Verification items for the finished model (mm, model axes). Round coordinates to 2 decimals unless told otherwise and drop trailing zeros. Order: outer loops, then holes, each group sorted by start corner. A loop starts at its lowest first (then second) coordinate and runs counter-clockwise, first axis right, second up. Notation, with made-up numbers: M -36,-33.5 L 10,-33.5 A24 cw 10,-21.5 Z; hole C -13,-29 d2. An arc over 180 degrees is marked long. One line per item, written item: value. Start each with the question number.
from build123d import *

# Parameters (mm, degrees)
F0_W     = 40
F0_H     = 50
F1_DEPTH = 3
F3_D     = 4.1
F4_D     = 5.1
F5_R     = 5


with BuildPart() as f1:
    # F0 (on Front) → F1 (new body)
    with BuildSketch(Plane.XZ):
        Rectangle(F0_W, F0_H)
    extrude(amount=-F1_DEPTH)

    # F3 (through all)
    with Locations(Plane.XZ):
        with Locations((0, 15.5), (0, -15.5)):
            Hole(F3_D / 2)

    # F4 (through all)
    with Locations(Plane.XZ):
        with Locations((-15, 0), (15, 0)):
            Hole(F4_D / 2)

    # F5
    f5_edges = [f1.edges().sort_by_distance(p)[0] for p in [
        (20, 1.5, 25),
        (20, 1.5, -25),
        (-20, 1.5, -25),
        (-20, 1.5, 25),
    ]]
    fillet(f5_edges, radius=F5_R)


solid = f1.part
1. Draft check along X on faces 1 (the face through (-12.452, 1.521, 0.112)), 2 (the face through (0, 1, 25)), 3 (the face through (18, 2, 24)). Enter one of: released by +X, released by -X, zero draft, split by the parting line, or undercut.
2. Scan lines: line 1 along Z through (x, y) = (0, 0.7); line 2 along Z through (x, y) = (-15, 0.6); line 3 along Z through (x, y) = (1, 1.45). Record each from-to range of solid material in increasing order.
3. Section check B-B (x = 0). Record the cut outline in (y, z).
4. Section check C-C (y = 2). Record the cut outline in (x, z).
5. Section check D-D (z = 15.5). Record the cut outline in (x, y).
6. Section check A-A (z = 0). Record the cut outline in (x, y), and give its area (3 significant figures).
Geometry check:
1. face 1: undercut
1. face 2: zero draft
1. face 3: released by +X
2. line 1: z = -25 to -17.55, -13.45 to 13.45, 17.55 to 25
2. line 2: z = -25 to -2.55, 2.55 to 25
2. line 3: z = -25 to -17.29, -13.71 to 13.71, 17.29 to 25
3. outline: M 0,-25 L 3,-25 L 3,-17.55 L 0,-17.55 Z; M 0,-13.45 L 3,-13.45 L 3,13.45 L 0,13.45 Z; M 0,17.55 L 3,17.55 L 3,25 L 0,25 Z
4. outline: M -20,-20 A5 ccw -15,-25 L 15,-25 A5 ccw 20,-20 L 20,20 A5 ccw 15,25 L -15,25 A5 ccw -20,20 Z; hole C -15,0 d5.1; hole C 0,-15.5 d4.1; hole C 0,15.5 d4.1; hole C 15,0 d5.1
5. outline: M -20,0 L -2.05,0 L -2.05,3 L -20,3 Z; M 2.05,0 L 20,0 L 20,3 L 2.05,3 Z
6. outline: M -20,0 L -17.55,0 L -17.55,3 L -20,3 Z; M -12.45,0 L 12.45,0 L 12.45,3 L -12.45,3 Z; M 17.55,0 L 20,0 L 20,3 L 17.55,3 Z
6. area: 89.4 mm²
